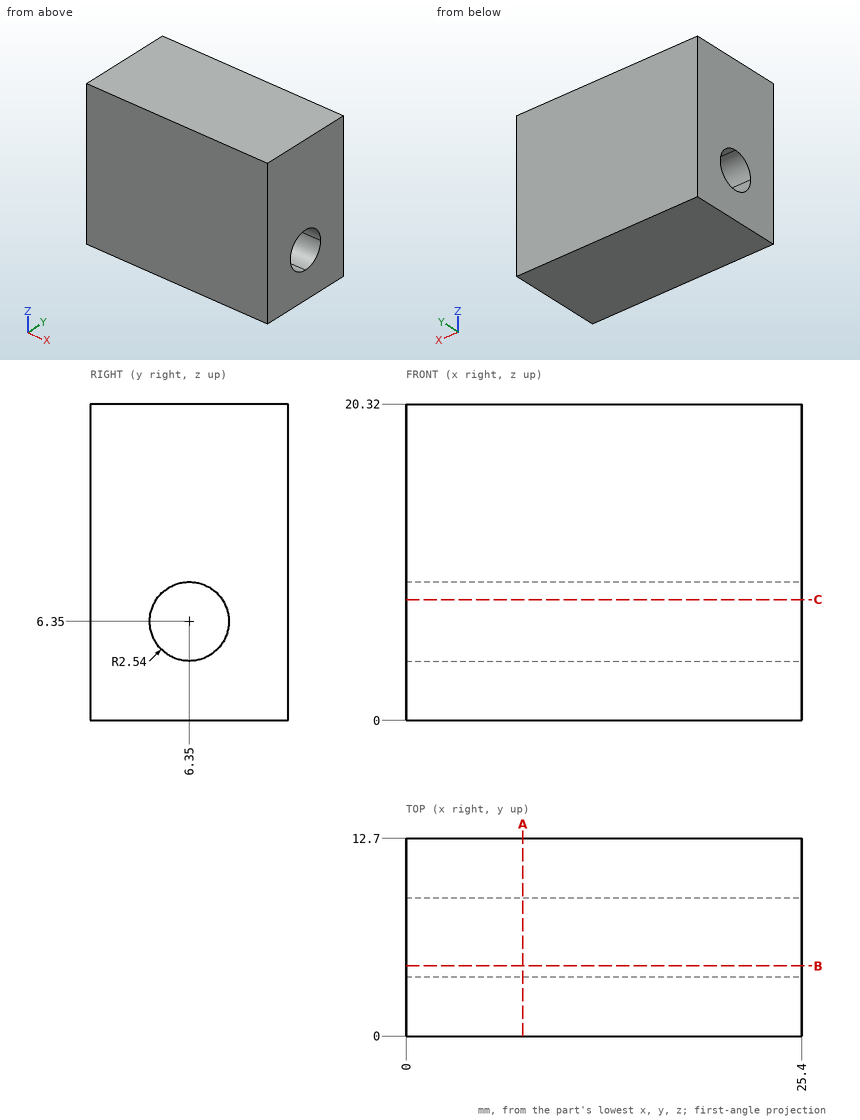
Geometry check sheet. Reference: drawing and pictorial views, mm from the part's lowest x, y, z. Round coordinates to 2 decimals unless told otherwise and drop trailing zeros. Write each loop counter-clockwise with the first axis right and the second up, starting at its lowest first coordinate (ties: lowest second). Pieces come first, ordered by that corner, then holes.
1. Scan lines: L1, parallel to Y at x = 6.5, z = 8; L2, parallel to Y at x = 13.5, z = 8.25; L3, parallel to Z at x = 13.25, y = 6.75. Record each from-to range of solid material in increasing order.
2. Section check B-B on y = 4.5. Enter the section's corners in (x, z), plus the area to 3 significant figures.
3. Section check C-C on z = 7.75. Enter the section's corners in (x, y).
4. Section check A-A on x = 7.5. Enter the section's corners in (y, z).
Answer:
1. L1: y = 0 to 4.42, 8.28 to 12.7
1. L2: y = 0 to 4.66, 8.04 to 12.7
1. L3: z = 0 to 3.84, 8.86 to 20.32
2. outline: (0, 0) - (25.4, 0) - (25.4, 4.61) - (0, 4.61) - close; (0, 8.09) - (25.4, 8.09) - (25.4, 20.32) - (0, 20.32) - close
2. area: 428 mm2
3. outline: (0, 0) - (25.4, 0) - (25.4, 4.23) - (0, 4.23) - close; (0, 8.47) - (25.4, 8.47) - (25.4, 12.7) - (0, 12.7) - close
4. outline: (0, 0) - (12.7, 0) - (12.7, 20.32) - (0, 20.32) - close; hole (3.81, 6.35) arc R2.54 ccw to (6.35, 3.81) arc R2.54 ccw to (8.89, 6.35) arc R2.54 ccw to (6.35, 8.89) arc R2.54 ccw to start
